Autodesk Inventor part; units mm, degrees
ref_plane "Work Plane1" through (0, 20, 0) normal (0, -1, 0) x (1, 0, 0)
ref_plane "Work Plane2" through (0, 228, 0) normal (0, 1, 0) x (1, 0, 0)
ref_plane "YZ Plane" through (0, 0, 0) normal (1, 0, 0) x (0, 1, 0)
sketch "Sketch1" plane through (0, 0, 0) normal (0, 1, 0) x (-1, 0, 0)
  circle A0 centre (0, 0) radius 158
  circle A1 centre (0, 0) radius 160
  dimension "d0" = 316
  dimension "d1" = 320
extrude "Extrusion1" add sketch "Sketch1" along normal blind 240 and the other way blind 40
ref_plane "Work Plane1" through (0, 20, 0) normal (0, -1, 0) x (1, 0, 0)
sketch "Sketch3" plane through (0, 20, 0) normal (0, -1, 0) x (1, 0, 0)
  circle A0 centre (0, 0) radius 158
  circle A1 centre (0, 0) radius 154
  dimension "d8" = 308
  dimension "d16" = 316
extrude "Extrusion3" add sketch "Sketch3" against normal blind 4
ref_plane "Work Plane2" through (0, 228, 0) normal (0, 1, 0) x (1, 0, 0)
sketch "Sketch4" plane through (0, 228, 0) normal (0, 1, 0) x (1, 0, 0)
  circle A0 centre (0, 0) radius 158
  circle A1 centre (0, 0) radius 154
  dimension "d12" = 316
  dimension "d13" = 308
extrude "Extrusion4" add sketch "Sketch4" along normal blind 4
sketch "Sketch5" plane through (0, 228, 0) normal (0, 1, 0) x (1, 0, 0)
  line L0 (159.9875, -2) -> (-159.9875, -2)
  circle A0 centre (0, 0) radius 160
  arc A1 (-159.9875, -2) -> (159.9875, -2) centre (0, 0) ccw
  dimension "d17" = 2
extrude "Extrusion5" cut sketch "Sketch5" against normal blind 144 contours A0 L0 picked at (22.9687, -49.4673)
sketch "Sketch6" plane through (0, 240, 0) normal (0, 1, 0) x (1, 0, 0)
  circle A0 centre (0, 0) radius 190
  dimension "d22" = 380
extrude "Extrusion6" add sketch "Sketch6" along normal blind 4
fillet "Fillet1" radius 4 1 edges at (-190, 244, 0)
sketch "Sketch7" plane through (0, -40, 0) normal (0, -1, 0) x (1, 0, 0)
  circle A0 centre (0, 0) radius 190
  dimension "d26" = 380
extrude "Extrusion7" add sketch "Sketch7" along normal blind 4
fillet "Fillet2" radius 4 1 edges at (-190, -40, 0)
properties part number "OuterCover" material "Aluminum 6061"
Can you work these out from the model? Positions are in its coordinate system, mm. A direction names the side the tool comes from. Round coordinates to 2 decimals unless told otherwise and drop trailing zeros. Write each loop counter-clockwise with the first axis right and the second up, starting at its lowest first coordinate (ties: lowest second). Pieces come first, ordered by that corner, then holes. Notation, with made-up numbers: M 45.25,12 L 92.25,12 A20 cw 92.25,35 Z; hole C 76.5,33 d4. An arc over 180 degrees is marked long. Use CSV: the item, a comma, the result in double quotes.
(1) I'm going to push flat-ended pins straight in: pin 1 (6 mm diameter, centred on y = 134, z = -62, fed in from +X); pin 2 (2 mm diameter, centred on x = 159.5, y = 182.5, fed in from +Z); pin 3 (8 mm diameter, centred on x = -98, y = 168, fed in from -Z). Where does each tip first touch, or does it pass through?
Check values:
pin 1,"x = 148.72"
pin 2,"z = 2"
pin 3,"z = -129.48"
(2) Imagine slicing it at A-A (y = 128). Write out the boundary of the cut face in (x, z).
Check values:
outline,"M -159.99,2 A160 ccw long 159.99,2 L 157.99,2 A158 cw long -157.99,2 Z"
(3) We'd pull the mould along Y, two halves only. Please class faces 1 (the flat face through (-3, -44, 3)), 2 (the flat face through (-3, 244, -3)), 3 (the flat face through (34, 20, -151)): +Y half, -Y half, draft (parallel to the pull), parting line (faces both ways), or undercut.
Check values:
face 1,"-Y half"
face 2,"+Y half"
face 3,"undercut"
(4) On a 3-axis mill with a long thin cutter (end or side, diameter ignored), from which of +Z, -Z, +X, -X, +Y, -Y can I reach the whole of each face in a straight line? I mean faces 4 (the cylindrical face through (20.568, 101.905, -156.655)), 5 (the flat face through (-131, 228, 83)), 6 (the flat face through (-24, 84, 157)). Say none if no direction works.
Check values:
face 4,"none"
face 5,"+Z"
face 6,"+Z, +X, -X"
(5) I need wall thicknesses on line 1 along Y through (x, z) = (-134.5, -102.5); line 2 along Z through (x, y) = (0, 229.2); line 3 along Z through (x, y) = (0, -11.5). Which ranges of each line are inside material? Lowest first, please.
Check values:
line 1,"-44 to -40, 240 to 244"
line 2,"-160 to -154, 154 to 160"
line 3,"-160 to -158, 158 to 160"
